Geometry check sheet. Reference: drawing and pictorial views, mm from the part's lowest x, y, z. A direction names the side the tool comes from. Round coordinates to 2 decimals unless told otherwise and drop trailing zeros. Loops run counter-clockwise (first coordinate to the right, second up) from the corner with the lowest first, then second, coordinate; pieces in that order, holes last. Notation, with made-up numbers: (36.5, -30) -> (82.5, -30) arc R22 ccw to (82.5, 5) -> close; hole circle Ø1 at (1.5, 8.25). An arc over 180 degrees is marked (long way). Use one line per item in the form item = value. Start each with the question number.
(1) Sectioned sample at A-A (z = 25.5). Record the cut outline in (x, y).
(2) Set-up check for the marked faces 1, 2, 3 and 4: record each of +Z, -Z, +X, -X, +Y, -Y from which the full face is reachable in a straight line by a thin tool's end or side.
(3) Sectioned sample at D-D (z = 6). Record the cut outline in (x, y), and give its area (3 significant figures).
(4) Sectioned sample at C-C (y = 5). Record the cut outline in (x, z).
(5) Go/stop test with flat-tipped pins: pin 1 (0.6 mm diameter, centred on y = 7, z = 1, fed in from +X); pin 2 (0.6 mm diameter, centred on x = 3, y = 0.5, fed in from -Z); pin 3 (3 mm diameter, centred on x = 2.5, z = 3.5, fed in from +Y). Record where each tip stops, or that it passes through.
(6) Sectioned sample at B-B (x = 2.5). Record the cut outline in (y, z), and give its area (3 significant figures).
(7) Material ranges on probe 1 along Y at (x, z) = (3, 0.3); probe 2 along X at (y, z) = (5, 0.6); probe 3 along Z at (x, y) = (2.95, 5), recorded low to high. Write a range as [from, to].
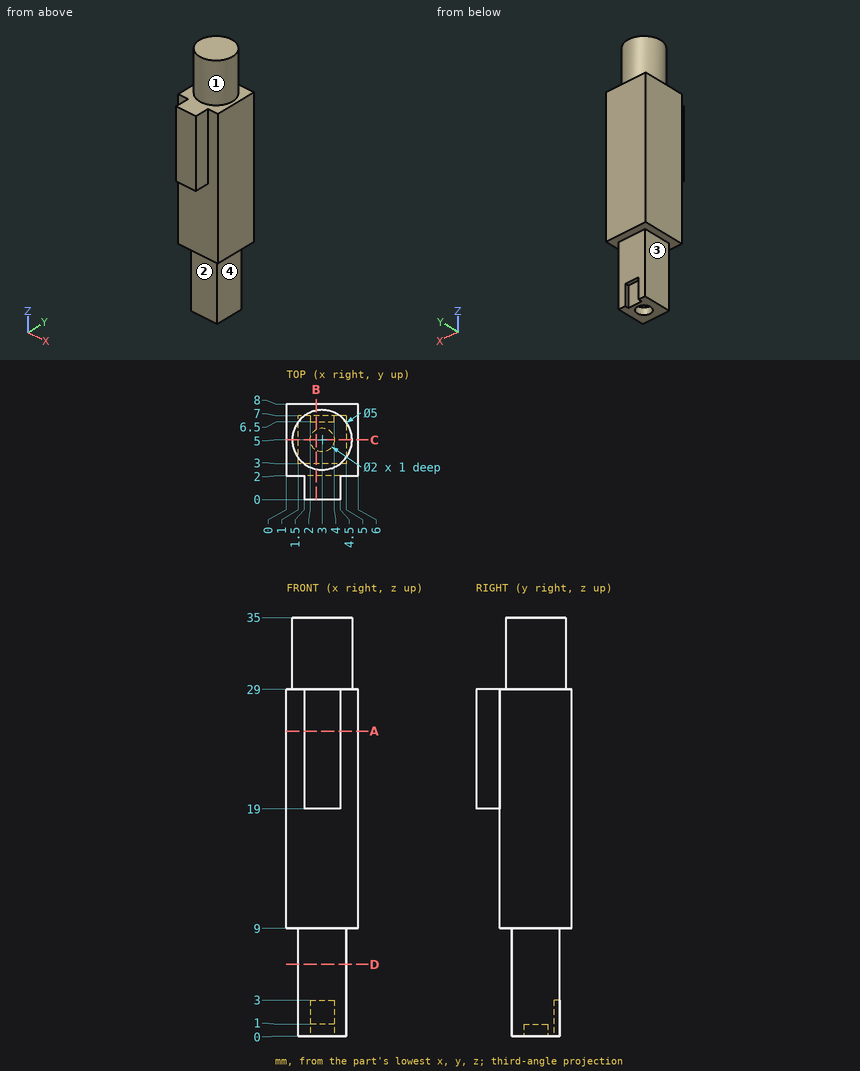
Checks:
q1.outline = (0, 2) -> (1.5, 2) -> (1.5, 0) -> (4.5, 0) -> (4.5, 2) -> (6, 2) -> (6, 8) -> (0, 8) -> close
q2.face_1 = +Z
q2.face_2 = -Z, +X, -X, -Y
q2.face_3 = -Z, -X, +Y, -Y
q2.face_4 = -Z, +X, +Y, -Y
q3.outline = (1, 3) -> (5, 3) -> (5, 7) -> (1, 7) -> close
q3.area = 16.0 mm2
q4.outline = (0, 9) -> (1, 9) -> (1, 0) -> (2, 0) -> (2, 1) -> (4, 1) -> (4, 0) -> (5, 0) -> (5, 9) -> (6, 9) -> (6, 29) -> (5.5, 29) -> (5.5, 35) -> (0.5, 35) -> (0.5, 29) -> (0, 29) -> close
q5.pin_1 = 5
q5.pin_2 = 19
q5.pin_3 = 7
q6.outline = (0, 19) -> (2, 19) -> (2, 9) -> (3, 9) -> (3, 0) -> (4.13, 0) -> (4.13, 1) -> (5.87, 1) -> (5.87, 0) -> (6.5, 0) -> (6.5, 3) -> (7, 3) -> (7, 9) -> (8, 9) -> (8, 29) -> (7.45, 29) -> (7.45, 35) -> (2.55, 35) -> (2.55, 29) -> (0, 29) -> close
q6.area = 202 mm2
q7.probe_1 = [3, 4], [6, 6.5]
q7.probe_2 = [1, 2], [4, 5]
q7.probe_3 = [1, 35]
